Geometry check sheet. Reference: the model listing, model coordinates, mm. Face numbers are marked on the shaded views. Coordinates: 2 decimals unless noted, no trailing zeros. Loops run counter-clockwise (first coordinate to the right, second up) from the corner with the lowest first, then second, coordinate; pieces in that order, holes last. Notation, with made-up numbers: (-26, -33) -> (33, -33) arc R14 cw to (33, -28) -> close; hole circle Ø1 at (6.5, 24.5). An arc over 180 degrees is marked (long way). Answer as a JSON object with one key per item and string values.
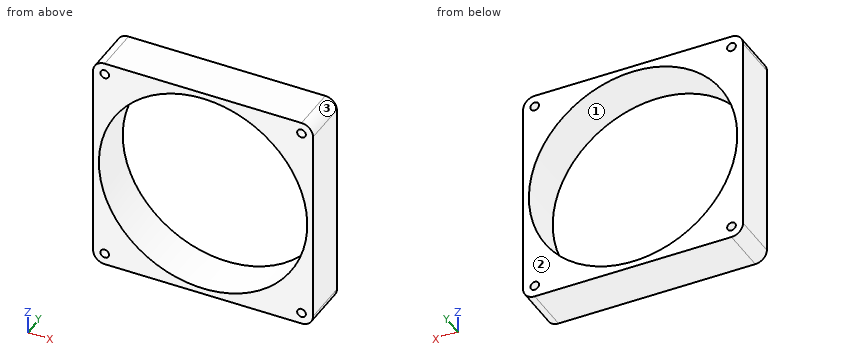
from build123d import *

# Parameters (mm, degrees)
SKETCH1_W           = 120.65
SKETCH1_H           = 120.65
BOSS_EXTRUDE1_DEPTH = 25.4
FILLET1_R           = 6.35
FILLET2_R           = 6.35
SKETCH2_R           = 2.38125
CUT_EXTRUDE1_DEPTH  = 137.199111623
SKETCH4_R           = 57.15
CUT_EXTRUDE2_DEPTH  = 25.4


with BuildPart() as part:
    # Sketch1 → Boss-Extrude1 (new body)
    with BuildSketch(Plane(origin=(0, 0, 0), x_dir=(1, 0, 0), z_dir=(0, 1, 0))):
        with Locations((27.733831169, -40.425584416)):
            Rectangle(SKETCH1_W, SKETCH1_H)
    extrude(amount=BOSS_EXTRUDE1_DEPTH)

    # Fillet1
    fillet1_edges = [part.edges().sort_by_distance(p)[0] for p in [
        (-32.591168831, 12.7, 100.750584416),
    ]]
    fillet(fillet1_edges, radius=FILLET1_R)

    # Fillet2
    fillet2_edges = [part.edges().sort_by_distance(p)[0] for p in [
        (-32.591168831, 12.7, -19.899415584),
        (88.058831169, 12.7, -19.899415584),
        (88.058831169, 12.7, 100.750584416),
    ]]
    fillet(fillet2_edges, radius=FILLET2_R)

    # Sketch2 → Cut-Extrude1 (cut, through all)
    with BuildSketch(Plane(origin=(0, 25.4, 0), x_dir=(1, 0, 0), z_dir=(0, 1, 0))):
        with Locations(Location((-26.241168831, -94.400584416, 0), (0, 0, 270))):
            Circle(SKETCH2_R)
        with Locations(Location((-26.241168831, 13.549415584, 0), (0, 0, 270))):
            Circle(SKETCH2_R)
        with Locations(Location((81.708831169, 13.549415584, 0), (0, 0, 270))):
            Circle(SKETCH2_R)
        with Locations(Location((81.708831169, -94.400584416, 0), (0, 0, 270))):
            Circle(SKETCH2_R)
    extrude(amount=-CUT_EXTRUDE1_DEPTH, mode=Mode.SUBTRACT)

    # Sketch4 → Cut-Extrude2 (cut)
    with BuildSketch(Plane(origin=(0, 25.4, 0), x_dir=(1, 0, 0), z_dir=(0, 1, 0))):
        with Locations(Location((27.733831169, -40.425584416, 0), (0, 0, 270))):
            Circle(SKETCH4_R)
    extrude(amount=-CUT_EXTRUDE2_DEPTH, mode=Mode.SUBTRACT)


solid = part.part
1. Section check A-A, the plane z = 21. Record the boundary of the cut face in (x, y), then the cut area to 3 significant figures.
Evaluation:
{"outline": "(-32.59, 0) -> (-26.01, 0) -> (-26.01, 25.4) -> (-32.59, 25.4) -> close; (81.48, 0) -> (88.06, 0) -> (88.06, 25.4) -> (81.48, 25.4) -> close", "area": "334 mm^2"}
2. Thickness scan on probe 1 along X at (y, z) = (7.25, 50); probe 2 along Z at (x, y) = (-24.5, 2.5) (3 decimals); probe 3 along X at (y, z) = (20, 41). Record the ranges inside material, lowest first. Write a range as from..to.
Evaluation:
{"probe 1": "x = -32.59..-28.61, 84.08..88.06", "probe 2": "z = -19.899..-15.174, -11.925..17.236, 63.615..92.776, 96.025..100.751", "probe 3": "x = -32.59..-29.41, 84.88..88.06"}
3. Section check C-C, the plane y = 23.25. Record the boundary of the cut face in (x, z).
Evaluation:
{"outline": "(-32.59, -13.55) arc R6.35 ccw to (-26.24, -19.9) -> (81.71, -19.9) arc R6.35 ccw to (88.06, -13.55) -> (88.06, 94.4) arc R6.35 ccw to (81.71, 100.75) -> (-26.24, 100.75) arc R6.35 ccw to (-32.59, 94.4) -> close; hole circle Ø114.3 at (27.73, 40.43); hole circle Ø4.76 at (-26.24, -13.55); hole circle Ø4.76 at (-26.24, 94.4); hole circle Ø4.76 at (81.71, -13.55); hole circle Ø4.76 at (81.71, 94.4)"}
4. Mould release check, pull along Z, two halves, no side actions. Record for the marked faces 1, 2 and 3: released by +Z, released by -Z, zero draft, split by the parting line, or undercut.
Evaluation:
{"face 1": "undercut", "face 2": "zero draft", "face 3": "released by +Z"}
5. Section check B-B, the plane x = 59. Record the boundary of the cut face in (y, z).
Evaluation:
{"outline": "(0, -19.9) -> (25.4, -19.9) -> (25.4, -7.41) -> (0, -7.41) -> close; (0, 88.26) -> (25.4, 88.26) -> (25.4, 100.75) -> (0, 100.75) -> close"}
